Geometry check sheet. Reference: drawing and pictorial views, mm from the part's lowest x, y, z. A direction names the side the tool comes from. Coordinates: 2 decimals unless noted, no trailing zeros. Write each loop counter-clockwise with the first axis right and the second up, starting at its lowest first coordinate (ties: lowest second). Pieces come first, ordered by that corner, then holes. Notation, with made-up numbers: (-33, -31) -> (-14, -31) arc R33 cw to (-14, 4) -> close; hole circle Ø3 at (-14.75, 7). An arc over 180 degrees is marked (long way). Use a Markdown table: item, result. Add a question column.
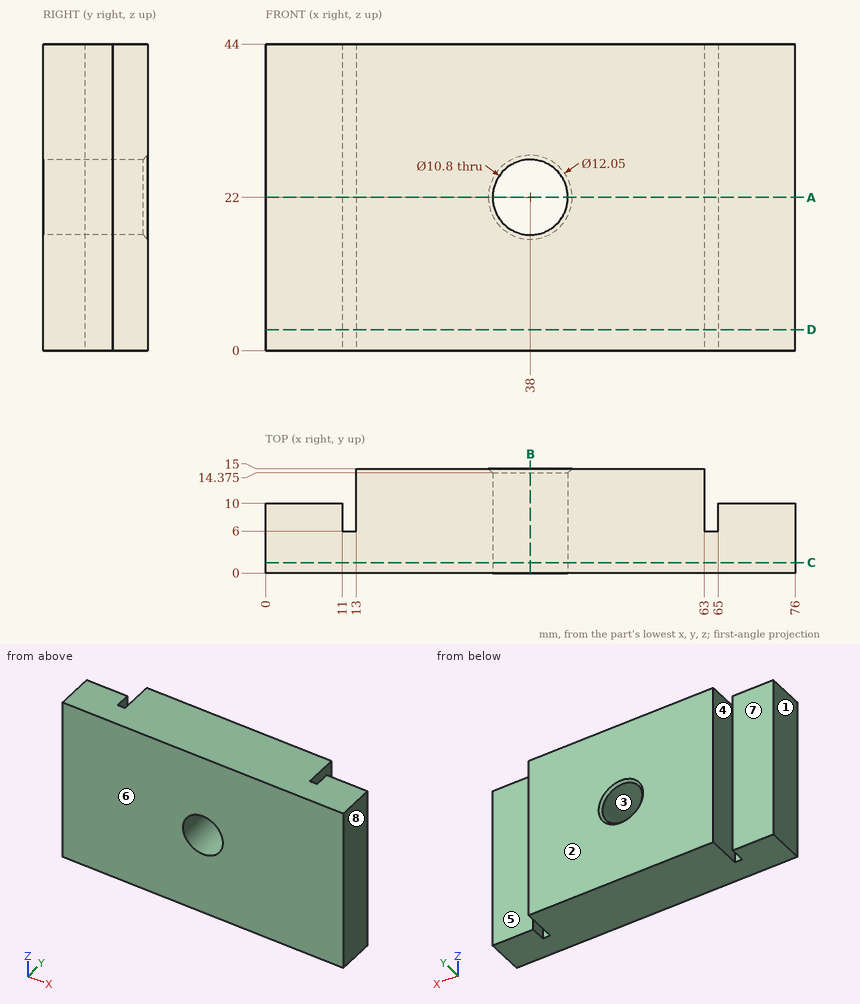
1) Cross-section at D-D on z = 3. Record the boundary of the cut face in (x, y).
2) Cross-section at A-A on z = 22. Record the boundary of the cut face in (x, y) (3 decimals), then the cut area to 3 significant figures.
3) Cross-section at B-B on x = 38. Record the boundary of the cut face in (y, z) (3 decimals).
4) Gauge pin test, flat end, axial feed: pin 1 (5.5 mm diameter, centred on x = 6.5, z = 11, fed in from +Y). Record the tip position at first contact, or that the pin passes through.
5) Cross-section at C-C on y = 1.5. Record the boundary of the cut face in (x, z), then the cut area to 3 significant figures.
6) Set-up check for the marked faces 4, 5, 6, 7 and 8: record each of +Z, -Z, +X, -X, +Y, -Y from which the full face is reachable in a straight line by a thin tool's end or side.
7) Release check for a two-part mould opening along X. For the marked faces 1, 2 and 3 record: released by +X, released by -X, zero draft, split by the parting line, or undercut.
8) Thickness scan on L1, parallel to X at y = 9, z = 38.5; L2, parallel to X at y = 8, z = 22; L3, parallel to Z at x = 38, y = 8.75. Record the ranges inside material, lowest first.
Returned:
| question | item | result |
|---|---|---|
| 1 | outline | (0, 0) -> (76, 0) -> (76, 10) -> (65, 10) -> (65, 6) -> (63, 6) -> (63, 15) -> (13, 15) -> (13, 6) -> (11, 6) -> (11, 10) -> (0, 10) -> close |
| 2 | outline | (0, 0) -> (32.6, 0) -> (32.6, 14.375) -> (31.975, 15) -> (13, 15) -> (13, 6) -> (11, 6) -> (11, 10) -> (0, 10) -> close; (43.4, 0) -> (76, 0) -> (76, 10) -> (65, 10) -> (65, 6) -> (63, 6) -> (63, 15) -> (44.025, 15) -> (43.4, 14.375) -> close |
| 2 | area | 832 mm² |
| 3 | outline | (0, 0) -> (15, 0) -> (15, 15.975) -> (14.375, 16.6) -> (0, 16.6) -> close; (0, 27.4) -> (14.375, 27.4) -> (15, 28.025) -> (15, 44) -> (0, 44) -> close |
| 4 | pin 1 | stops at y = 10 |
| 5 | outline | (0, 0) -> (76, 0) -> (76, 44) -> (0, 44) -> close; hole circle Ø10.8 at (38, 22) |
| 5 | area | 3,250 mm² |
| 6 | face 4 | +Z, -Z, +Y |
| 6 | face 5 | +Z, -Z, +X, +Y |
| 6 | face 6 | +Z, -Z, +X, -X, -Y |
| 6 | face 7 | +Z, -Z, -X, +Y |
| 6 | face 8 | +Z, -Z, +X, +Y, -Y |
| 7 | face 1 | released by -X |
| 7 | face 2 | zero draft |
| 7 | face 3 | undercut |
| 8 | L1 | x = 0 to 11, 13 to 63, 65 to 76 |
| 8 | L2 | x = 0 to 11, 13 to 32.6, 43.4 to 63, 65 to 76 |
| 8 | L3 | z = 0 to 16.6, 27.4 to 44 |
